Here's how the part is built. I have some questions about the finished solid (model axes, mm). A direction names the side the tool comes from. Give positions to 0.01 mm unless a question says otherwise; leave off trailing zeros. Order: outer loops, then holes, each group sorted by start corner. A loop starts at its lowest first (then second) coordinate and runs counter-clockwise, first axis right, second up. Notation, with made-up numbers: M 62.5,19 L 76.5,19 A17 ccw 76.5,37 Z; hole C 34,-37.5 d8. An arc over 180 degrees is marked long. Use CSV: the item, a comma, the result in double quotes. Start each with the question number.
```python
from build123d import *

# Parameters (mm, degrees)
F0_R     = 37.75
F0_R_2   = 1.5
F0_R_3   = 2
F1_DEPTH = 24
F0_R_4   = 1
F2_DEPTH = 23
F5_R     = 9
F5_R_2   = 8
F6_DEPTH = 25
F7_DEPTH = 15


# Not quite as in the source:
# - a fillet or chamfer that OpenCascade refuses, or shapes differently, is made with other operations: its cross-section is extruded or revolved along the edge and cut away or added


with BuildPart() as f1:
    # F0 (on Front) → F1 (new body)
    with BuildSketch(Plane.XZ):
        Circle(F0_R)
        with Locations((0, -31.5)):
            Circle(F0_R_2, mode=Mode.SUBTRACT)
        with Locations((26.2829258241, -12.2559295905)):
            Circle(F0_R_3, mode=Mode.SUBTRACT)
        with BuildLine():
            ThreePointArc((-24.2829258241, 12.2559295905), (-24.3303338098, 11.8230503626), (-24.47031025, 11.410693067))
            ThreePointArc((-24.47031025, 11.410693067), (-28.2355178383, 12.6888088184), (-24.2829258241, 12.2559295905))
        make_face(mode=Mode.SUBTRACT)
        with BuildLine():
            ThreePointArc((10.4598019781, 22.4311177292), (19.8581217638, 14.7721867038), (24.4913793103, 3.568590685))
            ThreePointArc((24.4913793103, 3.568590685), (30.8891705898, 5.4307950139), (34.75, 0))
            ThreePointArc((34.75, 0), (30.8891705898, -5.4307950139), (24.4913793103, -3.568590685))
            ThreePointArc((24.4913793103, -3.568590685), (0, -24.75), (-24.4913793103, -3.568590685))
            ThreePointArc((-24.4913793103, -3.568590685), (-34.75, 0), (-24.4913793103, 3.568590685))
            ThreePointArc((-24.4913793103, 3.568590685), (-23.7129158978, 7.0894371866), (-22.4311177292, 10.4598019781))
            ThreePointArc((-22.4311177292, 10.4598019781), (-8.4649985473, 23.2573923645), (10.4598019781, 22.4311177292))
        make_face(mode=Mode.SUBTRACT)
        with Locations((0, 31.5)):
            Circle(F0_R_2, mode=Mode.SUBTRACT)
    extrude(amount=F1_DEPTH)

    # F0 (on Front) → F2 (join)
    with BuildSketch(Plane.XZ):
        with BuildLine():
            ThreePointArc((-24.4913793103, 3.568590685), (-34.75, 0), (-24.4913793103, -3.568590685))
            ThreePointArc((-24.4913793103, -3.568590685), (-24.75, 0), (-24.4913793103, 3.568590685))
        make_face()
        with Locations((-29, 0)):
            Circle(F0_R_4, mode=Mode.SUBTRACT)
        with Locations((0, 31.5)):
            Circle(F0_R_2)
        with BuildLine():
            ThreePointArc((24.4913793103, 3.568590685), (24.6852601559, 1.7889748557), (24.75, 0))
            ThreePointArc((24.75, 0), (24.6852601559, -1.7889748557), (24.4913793103, -3.568590685))
            ThreePointArc((24.4913793103, -3.568590685), (30.8891705898, -5.4307950139), (34.75, 0))
            ThreePointArc((34.75, 0), (30.8891705898, 5.4307950139), (24.4913793103, 3.568590685))
        make_face()
        with Locations((29, 0)):
            Circle(F0_R_4, mode=Mode.SUBTRACT)
        with Locations((0, -31.5)):
            Circle(F0_R_2)
    extrude(amount=F2_DEPTH)

    # F3: chamfer of 3 on 2 edges, made by hand

    # F3_s1 → F3_t2 (revolve, cut)
    with BuildSketch(Plane.XY.offset(12.2559295905)):
        Polygon((-21.2829258241, -24), (-24.2829258241, -21), (-24.2829258241, -24), align=None)
    revolve(axis=Axis((-26.2829258241, -24, 12.2559295905), (0, -1, 0)), mode=Mode.SUBTRACT)

    # F3_s3 → F3_t4 (revolve, cut)
    with BuildSketch(Plane.XY.offset(-12.2559295905)):
        Polygon((31.2829258241, -24), (28.2829258241, -21), (28.2829258241, -24), align=None)
    revolve(axis=Axis((26.2829258241, -24, -12.2559295905), (0, -1, 0)), mode=Mode.SUBTRACT)

    # F5 (on offset) → F6 (cut)
    with BuildSketch(Plane.XY.offset(26.25)):
        with Locations((0, -12)):
            Circle(F5_R)
        with Locations((0, -12)):
            Circle(F5_R_2, mode=Mode.SUBTRACT)
    extrude(amount=F6_DEPTH, mode=Mode.SUBTRACT)

    # F5 (on offset) → F7 (cut, symmetric)
    with BuildSketch(Plane.XY.offset(26.25)):
        with Locations((0, -12)):
            Circle(F5_R_2)
    extrude(amount=F7_DEPTH, both=True, mode=Mode.SUBTRACT)


solid = f1.part
```
Q1. Imagine slicing it at B-B, the plane z = 21.5. Please give me the cut outline in (x, y), then the cut area to 3 significant figures.
Q2. I need wall thicknesses on line 1 (Z direction, x = 0, y = -23.2); line 2 (Z direction, x = 0.5, y = -22.5); line 3 (X direction, y = -9.25, z = 8.5). Which ranges of each line are inside material? Lowest first, please. Write a range as [from, to].
Q3. Imagine slicing it at C-C, the plane y = -12. Please give me the cut outline in (x, z), then the cut area to 3 significant figures.
Q4. Imagine slicing it at D-D, the plane z = 31.5. Please give me the cut outline in (x, y).
Q5. For P1, Ø4.5, axis at x = -26.28, z = 12.26, coming from the -Y side (3 decimals); P2, Ø8, axis at y = -4, z = -30, coming from the -X side; P3, Ø1.5, axis at x = 0.5, z = 32, coming from the -Y side, each with a flat end and sliding along its axis, tell me the tip position at first contact or that it passes through.
Q6. Imagine slicing it at A-A, the plane x = 0. Please give me the cut outline in (y, z).
Q7. For faces 5 (the face through (8, -24, -25)), 6 (the face through (7.63, -9.6, 25.17)), 7 (the face through (-34.747, -23.493, -0.199)), which set-ups out of +Z, -Z, +X, -X, +Y, -Y let a thin tool reach every point of the face, with its end or its side?
Q8. We'd pull the mould along Z, two halves only. Please class faces 1 (the face through (30, -23, -1)), 2 (the face through (0, -23, -31)), 3 (the face through (-8.183, -11.832, -36.852)), 4 (the face through (-9, -12, 32)): pulls with the +Z half, pulls with the -Z half, needs draft (parallel to the pull), parting line crosses it, or undercut.
Reply:
1,outline,"M -31.03,-24 L -12.26,-24 L -12.26,0 L -31.03,0 Z; M 12.26,-24 L 31.03,-24 L 31.03,0 L 12.26,0 Z"
1,area,"901 mm^2"
2,line 1,"z = [-37.75, -33], [-30, -24.75], [24.75, 30], [33, 37.75]"
2,line 2,"z = [-37.75, -24.74], [24.74, 37.75]"
2,line 3,"x = [-36.78, -23.24], [23.24, 36.78]"
3,outline,"M -9,26.25 L -9,36.66 A37.75 ccw long 9,36.66 L 9,26.25 L 8,26.25 L 8,23.42 A24.75 cw long -8,23.42 L -8,26.25 Z; hole C -29,0 d2; hole C -26.28,12.26 d4; hole C 26.28,-12.26 d4; hole C 29,0 d2"
3,area,"2,290 mm^2"
4,outline,"M -20.8,-24 L -1.5,-24 L -1.5,-23 L 1.5,-23 L 1.5,-24 L 20.8,-24 L 20.8,0 L -20.8,0 Z; hole C 0,-12 d18"
5,P1,"stops at y = -21.255"
5,P2,"stops at x = -27.37"
5,P3,"stops at y = -23"
6,outline,"M -24,-37.75 L 0,-37.75 L 0,-24.75 L -24,-24.75 L -24,-30 L -23,-30 L -23,-33 L -24,-33 Z; M -24,24.75 L -20,24.75 L -20,26.25 L -21,26.25 L -21,37.75 L -24,37.75 L -24,33 L -23,33 L -23,30 L -24,30 Z; M -4,24.75 L 0,24.75 L 0,37.75 L -3,37.75 L -3,26.25 L -4,26.25 Z"
7,face 5,"+Z, -Z, +X, -X, -Y"
7,face 6,"+Z"
7,face 7,"-Y"
8,face 1,"undercut"
8,face 2,"undercut"
8,face 3,"parting line crosses it"
8,face 4,"needs draft"
